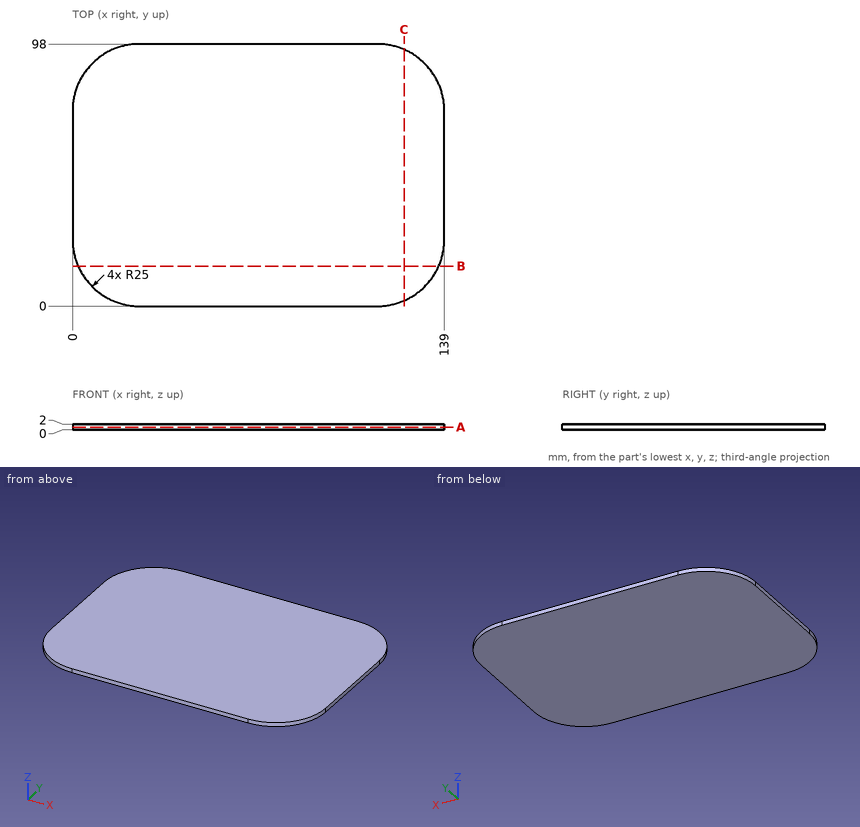
Geometry: see drawing. Coordinates: mm, zero at the bounding-box minimum. Coordinates: 2 decimals unless noted, no trailing zeros. Loops run counter-clockwise (first coordinate to the right, second up) from the corner with the lowest first, then second, coordinate; pieces in that order, holes last.
Q1. Cut plane A-A (z = 0.9). Output: boundary loops of the cut face in (x, y).
Q2. Material intervals for line 1 (Y direction, x = 133, z = 1.9); line 2 (Y direction, x = 129, z = 0.55); line 3 (X direction, y = 92.5, z = 0.5), sorted ascending.
Q3. Cut plane B-B (y = 15). Output: boundary loops of the cut face in (x, z), then the cut area to 3 significant figures.
Q4. Cut plane C-C (x = 124). Output: boundary loops of the cut face in (y, z), then the cut area to 3 significant figures.
Working result:
1. outline: (0, 25) arc R25 ccw to (25, 0) - (114, 0) arc R25 ccw to (139, 25) - (139, 73) arc R25 ccw to (114, 98) - (25, 98) arc R25 ccw to (0, 73) - close
2. line 1: y = 8.75 to 89.25
2. line 2: y = 5 to 93
2. line 3: x = 9.36 to 129.64
3. outline: (2.09, 0) - (136.91, 0) - (136.91, 2) - (2.09, 2) - close
3. area: 270 mm2
4. outline: (2.09, 0) - (95.91, 0) - (95.91, 2) - (2.09, 2) - close
4. area: 188 mm2
